The figure shows three views and two pictorial views of one solid part (mm, origin at its lowest corner). Answer the questions. A direction names the side the tool comes from. Give positions to 0.01 mm unless a question says otherwise; leave off trailing zeros. Write each loop counter-clockwise with the first axis right and the second up, starting at its lowest first coordinate (ties: lowest second). Pieces come first, ordered by that corner, then holes. Notation, with made-up numbers: (62.25, 42.5) - (91.25, 42.5) arc R11 ccw to (91.25, 49.5) - close; hole circle Ø2 at (-30, 21). An arc over 180 degrees is marked (long way). Write each question's results on one line, items separated by ' | '. Start each with the question number.
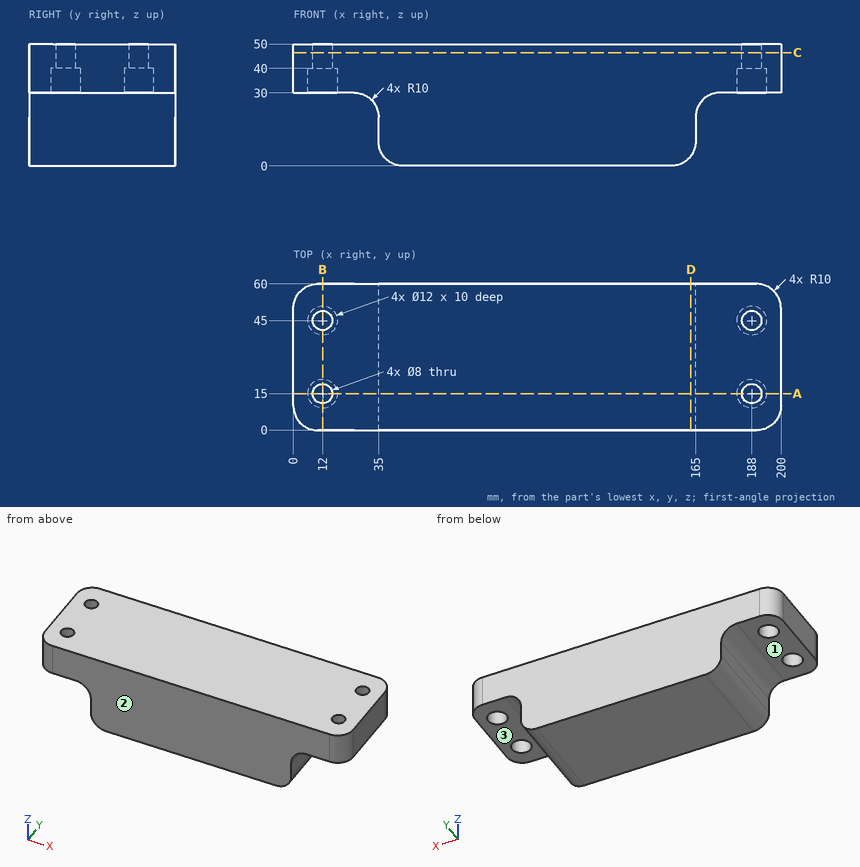
Q1. Consider L1, parallel to Y at x = 12, z = 43.5; L2, parallel to Y at x = 12, z = 37; L3, parallel to X at y = 42.5, z = 32. Determine where each line is inside the solid, lowest interval first.
Q2. A cutting plane is placed at D-D, the plane x = 163. Write down the section's boundary in (y, z).
Q3. A cutting plane is placed at C-C, the plane z = 46.5. Write down the section's boundary in (x, y).
Q4. A tool of negligible diameter and unlimited length cuts with its end or side. For the marked faces 1, 2 and 3, from which of +Z, -Z, +X, -X, +Y, -Y can it reach the whole face along a straight path? Write none if from no direction.
Q5. A cutting plane is placed at A-A, the plane y = 15. Write down the section's boundary in (x, z), and give its area (3 significant figures).
Q6. A cutting plane is placed at B-B, the plane x = 12. Write down the section's boundary in (y, z).
Q7. Given pin 1 (6 mm diameter, centred on x = 14, y = 47, fed in from -Z); pin 2 (11 mm diameter, centred on y = 36.5, z = 16.5, fed in from +X); pin 3 (8 mm diameter, centred on y = 35.5, z = 12.5, fed in from -X), each flat-ended and moving along its own axis, determine where each tip first touches the part or whether it passes through.
Result:
1) L1: y = 0 to 11, 19 to 41, 49 to 60 | L2: y = 0 to 9, 21 to 39, 51 to 60 | L3: x = 0 to 6.55, 17.45 to 182.55, 193.45 to 200
2) outline: (0, 4) - (60, 4) - (60, 50) - (0, 50) - close
3) outline: (0, 10) arc R10 ccw to (10, 0) - (190, 0) arc R10 ccw to (200, 10) - (200, 50) arc R10 ccw to (190, 60) - (10, 60) arc R10 ccw to (0, 50) - close; hole circle Ø8 at (12, 15); hole circle Ø8 at (12, 45); hole circle Ø8 at (188, 15); hole circle Ø8 at (188, 45)
4) face 1: -Z, -X, +Y, -Y | face 2: +Z, -Z, +X, -X, -Y | face 3: -Z, +X, +Y, -Y
5) outline: (0, 30) - (6, 30) - (6, 40) - (8, 40) - (8, 50) - (0, 50) - close; (16, 40) - (18, 40) - (18, 30) - (25, 30) arc R10 cw to (35, 20) - (35, 10) arc R10 ccw to (45, 0) - (155, 0) arc R10 ccw to (165, 10) - (165, 20) arc R10 cw to (175, 30) - (182, 30) - (182, 40) - (184, 40) - (184, 50) - (16, 50) - close; (192, 40) - (194, 40) - (194, 30) - (200, 30) - (200, 50) - (192, 50) - close | area: 7,500 mm2
6) outline: (0, 30) - (9, 30) - (9, 40) - (11, 40) - (11, 50) - (0, 50) - close; (19, 40) - (21, 40) - (21, 30) - (39, 30) - (39, 40) - (41, 40) - (41, 50) - (19, 50) - close; (49, 40) - (51, 40) - (51, 30) - (60, 30) - (60, 50) - (49, 50) - close
7) pin 1: stops at z = 40 | pin 2: stops at x = 165.2 | pin 3: stops at x = 35
